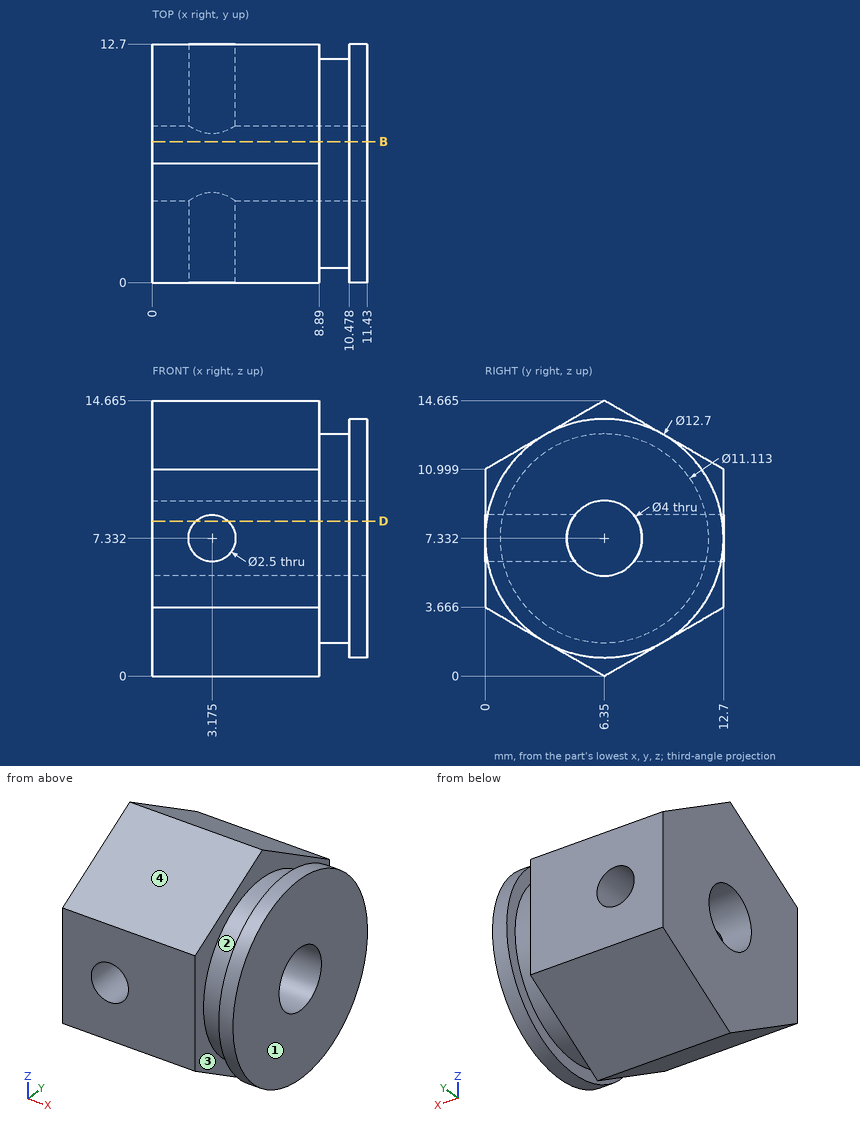
Design review of the part shown in the three views and the two pictorial views. Dimensions are in mm from the part's minimum x, y and z. Round coordinates to 2 decimals unless told otherwise and drop trailing zeros. Loops run counter-clockwise (first coordinate to the right, second up) from the corner with the lowest first, then second, coordinate; pieces in that order, holes last. Notation, with made-up numbers: M 73,88 L 91,88 A20 cw 91,94 Z; hole C -19,81.25 d6. An arc over 180 degrees is marked long. Put each result on its own line as item: value.
Q1. Consider section D-D, the plane z = 8.25. Give the boundary of the cut face in (x, y).
Result set:
outline: M 0,0 L 2.33,0 L 2.33,4.57 L 0,4.57 Z; M 0,8.13 L 2.33,8.13 L 2.33,12.7 L 0,12.7 Z; M 4.02,0 L 8.89,0 L 8.89,0.87 L 10.48,0.87 L 10.48,0.07 L 11.43,0.07 L 11.43,4.57 L 4.02,4.57 Z; M 4.02,8.13 L 11.43,8.13 L 11.43,12.63 L 10.48,12.63 L 10.48,11.83 L 8.89,11.83 L 8.89,12.7 L 4.02,12.7 Z
Q2. To check wall thickness, follow L1, parallel to X at y = 8.5, z = 2; L2, parallel to Z at x = 8.25, y = 5.75 (1 decimal); L3, parallel to Z at x = 1, y = 5.5 (1 decimal). State the ranges of each line that lie inside material, in increasing order.
Result set:
L1: x = 0 to 8.89, 10.48 to 11.43
L2: z = 0.3 to 5.4, 9.2 to 14.3
L3: z = 0.5 to 5.5, 9.1 to 14.2
Q3. Mouldability with a two-part tool opening along X and no side actions: class the marked faces 1, 2, 3 and 4 as released by +X, released by -X, zero draft, split by the parting line, or undercut.
Result set:
face 1: released by +X
face 2: undercut
face 3: undercut
face 4: zero draft
Q4. For pin 1 (1 mm diameter, centred on x = 8.5, z = 12.5, fed in from -Y) (1 decimal); pin 2 (2 mm diameter, centred on x = 3.18, z = 7.33, fed in from -Y); pin 3 (1 mm diameter, centred on x = 5.5, y = 5, fed in from +Z) (1 decimal), all flat-tipped, find the tip position at first contact; note any pin that passes through.
Result set:
pin 1: stops at y = 1.7
pin 2: passes through
pin 3: stops at z = 14.2
Q5. Consider section B-B, the plane y = 7.5. Give the boundary of the cut face in (x, z), then the cut area to 3 significant figures.
Result set:
outline: M 0,0.66 L 8.89,0.66 L 8.89,1.9 L 10.48,1.9 L 10.48,1.09 L 11.43,1.09 L 11.43,5.7 L 0,5.7 Z; M 0,8.97 L 11.43,8.97 L 11.43,13.58 L 10.48,13.58 L 10.48,12.77 L 8.89,12.77 L 8.89,14 L 0,14 Z
area: 110 mm²
